CAD build for the part. Positions are in the model's coordinates, mm. Face numbers are marked on the shaded views. A direction names the side the tool comes from. Give positions to 0.01 mm unless a question says otherwise; leave off trailing zeros. Order: outer loops, then holes, each group sorted by start corner. A loop starts at its lowest first (then second) coordinate and runs counter-clockwise, first axis right, second up. Notation, with made-up numbers: M 61,-38 L 116,-38 A13 ccw 116,-15 Z; hole C -5.75,39 d6. An arc over 180 degrees is marked long. Put each result on its own line as item: value. Start each with the question number.
1) Two-plate mould, pull along X, no slides. Class the marked faces 3, 4 and 5: released by +X, released by -X, zero draft, split by the parting line, or undercut.
2) Pin check, flat tips, straight feed: pin 1 (6 mm diameter, centred on y = 4, z = 6, fed in from -X); pin 2 (3 mm diameter, centred on y = -3.5, z = 6.5, fed in from -X); pin 3 (4 mm diameter, centred on y = -3.5, z = 9.5, fed in from +X). Stop position of each tip, or through.
3) Cut at D-D (x = -6). Write the cut outline in (y, z), and give its area (3 significant figures).
4) Cut at A-A (x = 0). Write the cut outline in (y, z).
5) Cut at C-C (z = 3). Write the cut outline in (x, y) (1 decimal).
6) Drill centre lines: line 1 (Z direction, x = -2.75, y = 6.75); line 2 (Y direction, x = 0, z = 5.5); line 3 (Y direction, x = 0, z = 8). Where is each one in solid material? Low to high. Write a range as [from, to].
7) Tool access for the marked faces 1 and 2: list every direction of +Z, -Z, +X, -X, +Y, -Y with a clear straight run to the whole face (end or side of a thin tool).
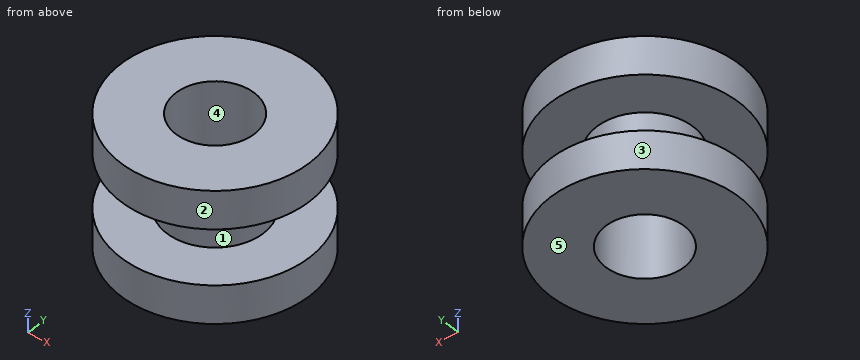
```python
from build123d import *

# Parameters (mm, degrees)
F0_R     = 4.064
F0_R_2   = 3.302
F1_DEPTH = 5.54482
F0_R_3   = 7.9375
F2_DEPTH = 3.2131


with BuildPart() as f1:
    # F0 (on Top) → F1 (new body)
    with BuildSketch(Plane.XY):
        Circle(F0_R)
        Circle(F0_R_2, mode=Mode.SUBTRACT)
    extrude(amount=F1_DEPTH)

    # F0 (on Top) → F2 (join)
    with BuildSketch(Plane.XY):
        Circle(F0_R_3)
        Circle(F0_R, mode=Mode.SUBTRACT)
    extrude(amount=F2_DEPTH)

    # F3: F1 across face


with BuildPart() as f1_1:
    add(f1.part)
    add(f1.part.mirror(Plane.XY.offset(5.54482)))


solid = f1_1.part
```
Solution:
1. face 3: split by the parting line
1. face 4: undercut
1. face 5: zero draft
2. pin 1: x = -7.76
2. pin 2: x = -7.39
2. pin 3: x = 7.79
3. outline: M -5.2,0 L 5.2,0 L 5.2,3.21 L -5.2,3.21 Z; M -5.2,7.88 L 5.2,7.88 L 5.2,11.09 L -5.2,11.09 Z
3. area: 66.8 mm²
4. outline: M -7.94,0 L -3.3,0 L -3.3,11.09 L -7.94,11.09 L -7.94,7.88 L -4.06,7.88 L -4.06,3.21 L -7.94,3.21 Z; M 3.3,0 L 7.94,0 L 7.94,3.21 L 4.06,3.21 L 4.06,7.88 L 7.94,7.88 L 7.94,11.09 L 3.3,11.09 Z
5. outline: C 0,0 d15.9; hole C 0,0 d6.6
6. line 1: [0, 3.21], [7.88, 11.09]
6. line 2: [-4.06, -3.3], [3.3, 4.06]
6. line 3: [-7.94, -3.3], [3.3, 7.94]
7. face 1: none
7. face 2: +Z, -Z
